Here's how the part is built. I have some questions about the finished solid (model axes, mm). Give positions to 0.01 mm unless a question says otherwise; leave off trailing zeros. Loops run counter-clockwise (first coordinate to the right, second up) from the corner with the lowest first, then second, coordinate; pieces in that order, holes last. Notation, with made-up numbers: (6, 6) - (16, 6) arc R25 cw to (16, 30) - close; hole circle Ø11 at (47.5, 70). An arc over 180 degrees is marked (long way). Use one line per item in the form item = value.
from build123d import *

# Parameters (mm, degrees)
BOSS_EXTRUDE1_DEPTH = 18
SKETCH2_R           = 5
SKETCH2_R_2         = 3.25
CUT_EXTRUDE1_DEPTH  = 19


with BuildPart() as part:
    # Sketch1 → Boss-Extrude1 (new body)
    with BuildSketch(Plane.XY):
        Polygon((-65.310735067, 157.079646018), (15.689264933, -242.920353982), (-65.310735067, -242.920353982), (-184.310735067, -242.920353982), (-184.310735067, 157.079646018), align=None)
    extrude(amount=BOSS_EXTRUDE1_DEPTH)

    # Sketch2 → Cut-Extrude1 (cut, through all)
    with BuildSketch(Plane(origin=(0, 0, 0), x_dir=(-1, 0, 0), z_dir=(0, 0, -1))):
        with Locations((84.310735067, 134.079646018)):
            Circle(SKETCH2_R)
        with Locations((161.310735067, 134.079646018)):
            Circle(SKETCH2_R)
        with Locations((143.060735067, 114.079646018)):
            Circle(SKETCH2_R_2)
        with Locations((143.060735067, 35.579646018)):
            Circle(SKETCH2_R_2)
        with Locations((143.060735067, -42.920353982)):
            Circle(SKETCH2_R_2)
        with Locations((143.060735067, -121.420353982)):
            Circle(SKETCH2_R_2)
        with Locations((143.060735067, -199.920353982)):
            Circle(SKETCH2_R_2)
        with Locations((169.310735067, -219.920353982)):
            Circle(SKETCH2_R)
        with Locations((3.968235067, -219.920353982)):
            Circle(SKETCH2_R)
    extrude(amount=-CUT_EXTRUDE1_DEPTH, mode=Mode.SUBTRACT)


solid = part.part
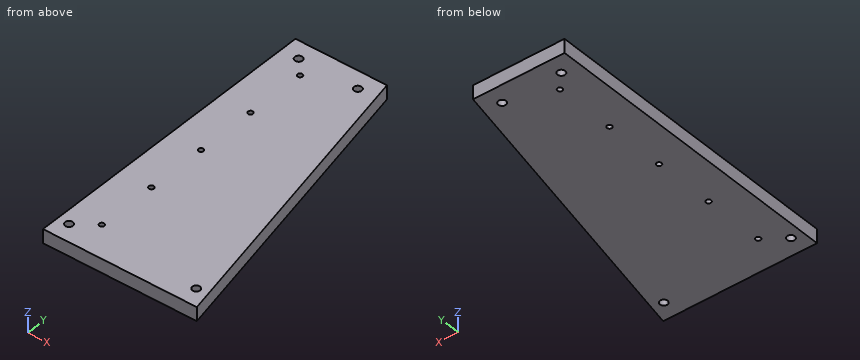
(1) If we section it at A-A (z = 9): Give the number of separate pieces and of enclosed holes in the cut face, plus the area to 3 significant figures.
Geometry says:
separate_pieces = 1
enclosed_holes = 9
area = 63,300 mm²
(2) If I drill on probe 1 along Y at (x, z) = (-158, 16.75); probe 2 along X at (y, z) = (38, 2.75); probe 3 along X at (y, z) = (121, 3.5), over which ranges is the centre line in solid material (lowest first)?
Geometry says:
probe_1 = -242.92 to 130.33, 137.83 to 157.08
probe_2 = -184.31 to -145.23, -140.89 to -41.2
probe_3 = -184.31 to -58
(3) If we section it at C-C (x = -26.5): List the corners of the cut face in (y, z) for me, plus the area to 3 significant figures.
Geometry says:
outline = (-242.92, 0) - (-34.58, 0) - (-34.58, 18) - (-242.92, 18) - close
area = 3,750 mm²
(4) If we section it at B-B (y = 18): List the corners of the cut face in (x, z) for me.
Geometry says:
outline = (-184.31, 0) - (-37.15, 0) - (-37.15, 18) - (-184.31, 18) - close
